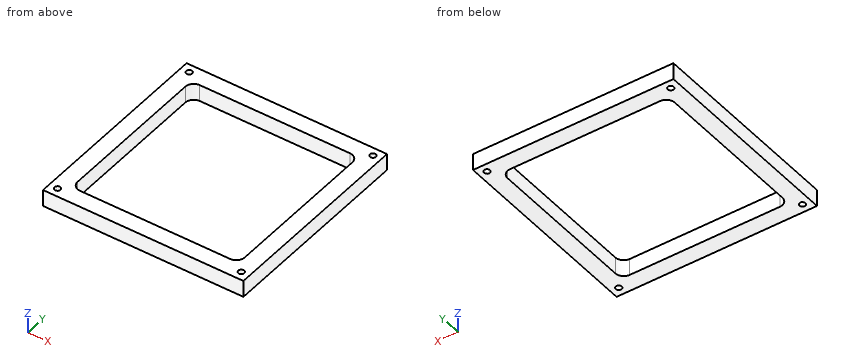
```python
from build123d import *

# Parameters (mm, degrees)
SKETCH1_W             = 152.4
SKETCH1_H             = 152.4
BOSS_EXTRUDE1_DEPTH   = 12.7
F_8_CLEARANCE_HOLE2_D = 4.4958
LPATTERN1_COUNT       = 2
LPATTERN1_PITCH       = 139.7
LPATTERN1_COUNT_DIR2  = 2
LPATTERN1_PITCH_DIR2  = 139.7


with BuildPart() as part:
    # Sketch1 → Boss-Extrude1 (new body)
    with BuildSketch(Plane.XY):
        with Locations((15.057340396, 3.848381836)):
            Rectangle(SKETCH1_W, SKETCH1_H)
        with BuildLine():
            Line((-42.092659604, 67.348381836), (72.207340396, 67.348381836))
            ThreePointArc((72.207340396, 67.348381836), (76.697468456, 65.488509896), (78.557340396, 60.998381836))
            Line((78.557340396, 60.998381836), (78.557340396, -53.301618164))
            ThreePointArc((78.557340396, -53.301618164), (76.697468456, -57.791746225), (72.207340396, -59.651618164))
            Line((72.207340396, -59.651618164), (-42.092659604, -59.651618164))
            ThreePointArc((-42.092659604, -59.651618164), (-46.582787665, -57.791746225), (-48.442659604, -53.301618164))
            Line((-48.442659604, -53.301618164), (-48.442659604, 60.998381836))
            ThreePointArc((-48.442659604, 60.998381836), (-46.582787665, 65.488509896), (-42.092659604, 67.348381836))
        make_face(mode=Mode.SUBTRACT)
    extrude(amount=BOSS_EXTRUDE1_DEPTH)

    # #8 Clearance Hole2 (through all)
    with Locations(Plane.XY.offset(12.7)):
        with Locations((-54.687907486, 73.795789856)):
            f_8_clearance_hole2 = Hole(F_8_CLEARANCE_HOLE2_D / 2)

    # LPattern1: 8 Clearance Hole2 2 × 2
    with Locations(*[(i * LPATTERN1_PITCH, -j * LPATTERN1_PITCH_DIR2, 0) for i in range(LPATTERN1_COUNT) for j in range(LPATTERN1_COUNT_DIR2) if (i, j) != (0, 0)]):
        add(f_8_clearance_hole2, mode=Mode.SUBTRACT)


solid = part.part
```
Read the model definition and answer for the solid it produces. Units are mm, in the model's axes. Coordinates: 2 decimals unless noted, no trailing zeros. Loops run counter-clockwise (first coordinate to the right, second up) from the corner with the lowest first, then second, coordinate; pieces in that order, holes last.
(1) The part is cut by section A-A (y = 46.5). Determine the outline of the cut face in (x, z), and give its area (3 significant figures).
Solution:
outline: (-61.14, 0) - (-48.44, 0) - (-48.44, 12.7) - (-61.14, 12.7) - close; (78.56, 0) - (91.26, 0) - (91.26, 12.7) - (78.56, 12.7) - close
area: 323 mm2
(2) The part is cut by section B-B (x = 8). Determine the outline of the cut face in (y, z).
Solution:
outline: (-72.35, 0) - (-59.65, 0) - (-59.65, 12.7) - (-72.35, 12.7) - close; (67.35, 0) - (80.05, 0) - (80.05, 12.7) - (67.35, 12.7) - close
(3) The part is cut by section C-C (z = 2.25). Determine the outline of the cut face in (x, y).
Solution:
outline: (-61.14, -72.35) - (91.26, -72.35) - (91.26, 80.05) - (-61.14, 80.05) - close; hole circle Ø4.5 at (-54.69, -65.9); hole circle Ø4.5 at (-54.69, 73.8); hole (-48.44, -53.3) arc R6.35 ccw to (-42.09, -59.65) - (72.21, -59.65) arc R6.35 ccw to (78.56, -53.3) - (78.56, 61) arc R6.35 ccw to (72.21, 67.35) - (-42.09, 67.35) arc R6.35 ccw to (-48.44, 61) - close; hole circle Ø4.5 at (85.01, -65.9); hole circle Ø4.5 at (85.01, 73.8)
(4) Consider line 1 along X through (y, z) = (21, 9); line 2 along Y through (x, z) = (32, 8.75); line 3 along X through (y, z) = (-58, 1.75). Determine where each line is inside the solid, lowest interval first.
Solution:
line 1: x = -61.14 to -48.44, 78.56 to 91.26
line 2: y = -72.35 to -59.65, 67.35 to 80.05
line 3: x = -61.14 to -46.36, 76.48 to 91.26
